The model under review builds one solid part; all positions refer to its coordinate system, in mm. A direction names the side the tool comes from. Round coordinates to 2 decimals unless told otherwise and drop trailing zeros. Order: outer loops, then holes, each group sorted by start corner. A loop starts at its lowest first (then second) coordinate and runs counter-clockwise, first axis right, second up.
1) Consider section B-B (x = 151.54). Give the boundary of the cut face in (y, z), then the cut area to 3 significant figures.
2) Machinability: for faces 1 (the face through (79, 5, -77)), 2 (the face through (30, 13, 75.8)), 3 (the face through (165.62, 7.57, -6.93)), 4 (the face through (-5, 5, 76.6)), 5 (the face through (-5, 9, 84.489)), which of the approach directions +Z, -Z, +X, -X, +Y, -Y give a long, thin tool a straight path to every point of the face, cutting with its end or side? Answer none if there is none.
3) Mouldability with a two-part tool opening along Z and no side actions: class faces 6 (the face through (-5, 5, 80.4)), 7 (the face through (87, 0, -1)), 8 (the face through (56, 13, -75.8)) as pulls with the +Z half, pulls with the -Z half, needs draft (parallel to the pull), parting line crosses it, or undercut.
4) Consider section C-C (z = -48.5). Give the boundary of the cut face in (x, y), then the cut area to 3 significant figures.
5) Consider section D-D (x = 10.5). Give the boundary of the cut face in (y, z), then the cut area to 3 significant figures.
6) Consider section A-A (z = 5.5). Give the boundary of the cut face in (x, y), then the cut area to 3 significant figures.
7) Clearance check with flat-ended pins moving along their axes: P1, Ø2, axis at x = 57, z = -78.5, coming from the +Y side; P2, Ø1.5, axis at y = 8, z = -10.5, coming from the -X side; P3, Ø2.5, axis at y = 12, z = -74.5, coming from the -X side. State where each tip first meets the part, or that it passes through.
8) To check wall thickness, follow L1, parallel to Z at x = 58, y = 12.5; L2, parallel to X at y = 4, z = 78.05; L3, parallel to X at y = 1.85, z = 78.05. State the ranges of each line that lie inside material, in increasing order.
from build123d import *

# Parameters (mm, degrees)
SKETCH1_W           = 159.54
SKETCH1_H           = 145
BOSS_EXTRUDE1_DEPTH = 3
BOSS_EXTRUDE2_DEPTH = 15
CUT_EXTRUDE1_DEPTH  = 3
CUT_EXTRUDE2_DEPTH  = 2
CUT_EXTRUDE3_DEPTH  = 12
CUT_EXTRUDE4_DEPTH  = 12
SKETCH8_R           = 1.1
SKETCH8_R_2         = 1.35
BOSS_EXTRUDE3_DEPTH = 10
BOSS_EXTRUDE5_DEPTH = 10
FILLET3_R           = 5
FILLET4_R           = 5
SKETCH10_R          = 1.325
CUT_EXTRUDE5_DEPTH  = 17
SKETCH12_R          = 3
CUT_EXTRUDE6_DEPTH  = 5
SKETCH13_R          = 6.25
CUT_EXTRUDE7_DEPTH  = 1


with BuildPart() as part:
    # Sketch1 → Boss-Extrude1 (new body)
    with BuildSketch(Plane(origin=(0, 0, 0), x_dir=(1, 0, 0), z_dir=(0, 1, 0))):
        with Locations((79.77, 0)):
            Rectangle(SKETCH1_W, SKETCH1_H)
    extrude(amount=BOSS_EXTRUDE1_DEPTH)

    # Sketch3 → Boss-Extrude2 (add)
    with BuildSketch(Plane(origin=(0, 0, 0), x_dir=(1, 0, 0), z_dir=(0, 1, 0))):
        Polygon((0, 72.5), (0, 84.5), (171.54, 84.5), (171.54, -84.5), (0, -84.5), (0, -72.5), (159.54, -72.5), (159.54, 72.5), align=None)
    extrude(amount=BOSS_EXTRUDE2_DEPTH)

    # Sketch4 → Cut-Extrude1 (cut)
    with BuildSketch(Plane(origin=(0, 15, 0), x_dir=(1, 0, 0), z_dir=(0, 1, 0))):
        Polygon((45.75, 75.8), (45.75, 72.5), (39.45, 72.5), (39.45, 75.8), (14.6, 75.8), (14.6, 80.3), (70.6, 80.3), (70.6, 75.8), align=None)
        Polygon((120.64, 75.8), (120.64, 72.5), (114.34, 72.5), (114.34, 75.8), (89.49, 75.8), (89.49, 80.3), (145.49, 80.3), (145.49, 75.8), align=None)
        Polygon((145.49, -75.8), (120.64, -75.8), (120.64, -72.5), (114.34, -72.5), (114.34, -75.8), (89.49, -75.8), (89.49, -80.3), (145.49, -80.3), align=None)
        Polygon((70.6, -75.8), (45.75, -75.8), (45.75, -72.5), (39.45, -72.5), (39.45, -75.8), (14.6, -75.8), (14.6, -80.3), (70.6, -80.3), align=None)
        Polygon((159.54, -38.5), (162.84, -38.5), (162.84, -18.15), (167.34, -18.15), (167.34, -65.15), (162.84, -65.15), (162.84, -44.8), (159.54, -44.8), align=None)
        Polygon((159.54, 40.6), (162.84, 40.6), (162.84, 65.45), (167.34, 65.45), (167.34, 9.45), (162.84, 9.45), (162.84, 34.3), (159.54, 34.3), align=None)
    extrude(amount=-CUT_EXTRUDE1_DEPTH, mode=Mode.SUBTRACT)

    # Sketch5 → Cut-Extrude2 (cut)
    with BuildSketch(Plane(origin=(0, 12, 0), x_dir=(1, 0, 0), z_dir=(0, 1, 0))):
        Polygon((39.45, -72.5), (39.45, -75.8), (33.99806762, -75.8), (33.99806762, -80.3), (51.20193238, -80.3), (51.20193238, -75.8), (45.75, -75.8), (45.75, -72.5), align=None)
        Polygon((114.34, -75.8), (108.704865037, -75.8), (108.704865037, -80.3), (126.275134963, -80.3), (126.275134963, -75.8), (120.64, -75.8), (120.64, -72.5), (114.34, -72.5), align=None)
        Polygon((120.64, 72.5), (114.34, 72.5), (114.34, 75.8), (108.704865037, 75.8), (108.704865037, 80.3), (126.308635122, 80.3), (126.308635122, 75.8), (120.64, 75.8), align=None)
        Polygon((45.75, 72.5), (39.45, 72.5), (39.45, 75.8), (34.110302497, 75.8), (34.110302497, 80.3), (51.089697503, 80.3), (51.089697503, 75.8), (45.75, 75.8), align=None)
        Polygon((159.54, -44.8), (159.54, -38.5), (162.84, -38.5), (162.84, -32.205861204), (167.34, -32.205861204), (167.34, -51.094138796), (162.84, -51.094138796), (162.84, -44.8), align=None)
        Polygon((159.54, 40.6), (162.84, 40.6), (162.84, 44.579740263), (167.34, 44.579740263), (167.34, 30.320259737), (162.84, 30.320259737), (162.84, 34.3), (159.54, 34.3), align=None)
    extrude(amount=-CUT_EXTRUDE2_DEPTH, mode=Mode.SUBTRACT)

    # Sketch6 → Cut-Extrude3 (cut)
    with BuildSketch(Plane(origin=(171.54, 0, 0), x_dir=(0, 0, -1), z_dir=(1, 0, 0))):
        with BuildLine():
            Line((-12.45, 10.5), (3.93, 10.5))
            ThreePointArc((3.93, 10.5), (6.93, 7.5), (3.93, 4.5))
            Line((3.93, 4.5), (-12.45, 4.5))
            ThreePointArc((-12.45, 4.5), (-15.45, 7.5), (-12.45, 10.5))
        make_face()
    extrude(amount=-CUT_EXTRUDE3_DEPTH, mode=Mode.SUBTRACT)

    # Sketch7 → Cut-Extrude4 (cut)
    with BuildSketch(Plane(origin=(0, 0, -84.5), x_dir=(-1, 0, 0), z_dir=(0, 0, -1))):
        with BuildLine():
            Line((-4.24, 10.6343), (12.14, 10.6343))
            ThreePointArc((12.14, 10.6343), (15.14, 7.6343), (12.14, 4.6343))
            Line((12.14, 4.6343), (-4.24, 4.6343))
            ThreePointArc((-4.24, 4.6343), (-7.24, 7.6343), (-4.24, 10.6343))
        make_face()
    extrude(amount=-CUT_EXTRUDE4_DEPTH, mode=Mode.SUBTRACT)

    # Sketch8 → Boss-Extrude3 (add)
    with BuildSketch(Plane.ZY):
        with Locations(Location((-78.5, 12.81715, 0), (0, 0, 180))):
            Circle(SKETCH8_R)
        with Locations(Location((-78.5, 2.328843142, 0), (0, 0, 180))):
            Circle(SKETCH8_R_2)
    extrude(amount=BOSS_EXTRUDE3_DEPTH)

    # Sketch9 → Boss-Extrude5 (add)
    with BuildSketch(Plane.ZY):
        Polygon((76.6, 14.98895691), (80.4, 14.98895691), (80.4, 10.9), (84.489160504, 10.9), (84.489160504, 7.1), (80.4, 7.1), (80.4, 3.01104309), (76.6, 3.01104309), (76.6, 7.100000004), (72.511375857, 7.100000004), (72.511117499, 10.899999996), (76.6, 10.899999996), align=None)
    extrude(amount=BOSS_EXTRUDE5_DEPTH)

    # Fillet3
    fillet3_edges = [part.edges().sort_by_distance(p)[0] for p in [
        (171.54, 7.5, 84.5),
    ]]
    fillet(fillet3_edges, radius=FILLET3_R)

    # Fillet4
    fillet4_edges = [part.edges().sort_by_distance(p)[0] for p in [
        (171.54, 7.5, -84.5),
    ]]
    fillet(fillet4_edges, radius=FILLET4_R)

    # Sketch10 → Cut-Extrude5 (cut)
    with BuildSketch(Plane.XZ):
        with Locations(Location((80.0525, 78.05, 0), (0, 0, 270))):
            Circle(SKETCH10_R)
        with Locations(Location((164.807766953, 77.767766953, 0), (0, 0, 270))):
            Circle(SKETCH10_R)
        with Locations(Location((164.807766953, -77.767766953, 0), (0, 0, 270))):
            Circle(SKETCH10_R)
        with Locations(Location((80.0525, -78.05, 0), (0, 0, 270))):
            Circle(SKETCH10_R)
    extrude(amount=-CUT_EXTRUDE5_DEPTH, mode=Mode.SUBTRACT)

    # Sketch12 → Cut-Extrude6 (cut)
    with BuildSketch(Plane(origin=(0, 0, 0), x_dir=(-1, 0, 0), z_dir=(0, -1, 0))):
        with Locations(Location((-80.0525, -78.05, 0), (0, 0, 90))):
            Circle(SKETCH12_R)
        with Locations(Location((-164.807766953, -77.767766953, 0), (0, 0, 90))):
            Circle(SKETCH12_R)
        with Locations(Location((-164.807766953, 77.767766953, 0), (0, 0, 90))):
            Circle(SKETCH12_R)
        with Locations(Location((-80.0525, 78.05, 0), (0, 0, 90))):
            Circle(SKETCH12_R)
    extrude(amount=-CUT_EXTRUDE6_DEPTH, mode=Mode.SUBTRACT)

    # Sketch13 → Cut-Extrude7 (cut)
    with BuildSketch(Plane.XZ):
        with Locations(Location((151.54, 64.5, 0), (0, 0, 270))):
            Circle(SKETCH13_R)
        with Locations(Location((151.54, -64.5, 0), (0, 0, 270))):
            Circle(SKETCH13_R)
    extrude(amount=-CUT_EXTRUDE7_DEPTH, mode=Mode.SUBTRACT)


solid = part.part
Answer below:
1. outline: (0, -84.5) - (15, -84.5) - (15, -72.5) - (3, -72.5) - (3, 72.5) - (15, 72.5) - (15, 84.5) - (0, 84.5) - (0, 70.75) - (1, 70.75) - (1, 58.25) - (0, 58.25) - (0, -58.25) - (1, -58.25) - (1, -70.75) - (0, -70.75) - close
1. area: 770 mm2
2. face 1: -Y
2. face 2: +Y
2. face 3: +X, -X
2. face 4: -X, -Y
2. face 5: +Z, +X, -X, +Y, -Y
3. face 6: pulls with the +Z half
3. face 7: needs draft
3. face 8: undercut
4. outline: (0, 0) - (171.54, 0) - (171.54, 15) - (167.34, 15) - (167.34, 12) - (162.84, 12) - (162.84, 15) - (159.54, 15) - (159.54, 3) - (0, 3) - close
4. area: 645 mm2
5. outline: (0, -84.5) - (15, -84.5) - (15, -72.5) - (3, -72.5) - (3, 72.5) - (15, 72.5) - (15, 84.5) - (0, 84.5) - close
5. area: 795 mm2
6. outline: (0, 0) - (171.54, 0) - (171.54, 4.5) - (159.54, 4.5) - (159.54, 3) - (0, 3) - close; (159.54, 10.5) - (171.54, 10.5) - (171.54, 15) - (159.54, 15) - close
6. area: 587 mm2
7. P1: stops at y = 12
7. P2: stops at x = 159.54
7. P3: stops at x = 0
8. L1: z = -84.5 to -80.3, -75.8 to -72.5, 72.5 to 75.8, 80.3 to 84.5
8. L2: x = -10 to 77.05, 83.05 to 161.82, 167.79 to 171.54
8. L3: x = 0 to 77.05, 83.05 to 161.82, 167.79 to 171.54
